Can you work these out from the model? Positions are in its coordinate system, mm. A direction names the side the tool comes from. Give positions to 0.01 mm unless a question says otherwise; leave off trailing zeros. Order: outer loops, then holes, each group sorted by start corner. A loop starts at its lowest first (then second) coordinate and runs counter-clockwise, first axis right, second up.
Item 1: I'm going to push flat-ended pins straight in: pin 1 Ø2.5 at (x, y) = (86, -43) entering from +Z; pin 2 Ø6.5 at (x, y) = (-95.5, 14.5) entering from +Z; pin 3 Ø1.5 at (x, z) = (30, 2) entering from -Y; pin 4 Ø1.8 at (x, y) = (30, -20) entering from +Z. Where does each tip first touch, or does it pass through?
Item 2: Which directions (+Z, -Z, +X, -X, +Y, -Y) give clear straight access to the entire face, cutting with the end or side of a thin tool? Please do faces 1 (the flat face through (-1, 1, 5)), 2 (the cylindrical face through (-81.095, 45.867, 3.479)), 3 (the flat face through (-47, -35, 3)), 4 (the flat face through (29, -57, 3)), 5 (the cylindrical face through (9.905, -29.867, 1.521)).
Item 3: If I drill on line 1 along X through (y, z) = (29, 1.2); line 2 along Y through (x, z) = (-72, 3.15); line 3 along X through (y, z) = (-15, 3.05), over which ranges is the centre line in solid material (lowest first)?
Item 4: I want a section at A-A, the plane x = -43.5. Write out the boundary of the cut face in (y, z), then the cut area to 3 significant figures.
Item 5: If we mould it in two halves opening along Y, with no side actions, what happens to faces 6 (the flat face through (-40, -60, 2)), 7 (the flat face through (-17, 31, 3)), 8 (the flat face through (70, 60, 2))? For each: +Y half, -Y half, draft (parallel to the pull), parting line (faces both ways), or undercut.
Autodesk Fusion 360 part; units mm, degrees
sketch "Sketch1" plane through (0, 0, 0) normal (0, 0, 1) x (1, 0, 0)
  line L0 (-105, 60) -> (105, 60)
  line L1 (105, 60) -> (105, -60)
  line L2 (105, -60) -> (-105, -60)
  line L3 (-105, -60) -> (-105, 60)
  line L4 (-105, 60) -> (105, -60) construction
  line L5 (105, 60) -> (-105, -60) construction
  dimension "d1" = 210
  dimension "d2" = 120
extrude "Extrude1" add sketch "Sketch1" along normal blind 5
sketch "Sketch2" plane through (0, 0, 5) normal (0, 0, 1) x (1, 0, 0)
  line L0 (-105, -60) -> (105, -60)
  line L1 (105, -60) -> (105, 60)
  line L2 (105, 60) -> (-105, 60)
  line L3 (-105, 60) -> (-105, -60)
  line L4 (0, 60) -> (0, -60) construction
  line L5 (105, 0) -> (-105, 0) construction
  line L6 (-75, 35) -> (-90, 35)
  line L7 (-90, 35) -> (-90, 38)
  line L8 (-90, 38) -> (-75, 38)
  line L9 (-75, 38) -> (-75, 35)
  line L10 (-75, 35) -> (-90, 38) construction
  line L11 (-90, 35) -> (-75, 38) construction
  line L12 (-55, 38) -> (-40, 38)
  line L13 (-40, 38) -> (-40, 35)
  line L14 (-40, 35) -> (-55, 35)
  line L15 (-55, 35) -> (-55, 38)
  line L16 (-55, 38) -> (-40, 35) construction
  line L17 (-40, 38) -> (-55, 35) construction
  line L18 (-40, -38) -> (-40, -35)
  line L19 (-55, -38) -> (-40, -35) construction
  line L20 (-40, -35) -> (-55, -35)
  line L21 (-55, -35) -> (-55, -38)
  line L22 (-55, -38) -> (-40, -38)
  line L23 (-40, -38) -> (-55, -35) construction
  line L24 (-75, -38) -> (-75, -35)
  line L25 (-90, -38) -> (-75, -38)
  line L26 (-90, -35) -> (-75, -38) construction
  line L27 (-75, -35) -> (-90, -38) construction
  line L28 (-75, -35) -> (-90, -35)
  line L29 (-90, -35) -> (-90, -38)
  point P0 (-85, 45)
  point P1 (85, 45)
  point P2 (30, 20)
  point P3 (19, 29)
  point P4 (6, 29)
  point P5 (-17, 29)
  point P6 (-30, 29)
  point P7 (-82.5, 36.5)
  point P8 (-47.5, 36.5)
  point P9 (-82.5, 36.5)
  point P10 (-47.5, 36.5)
  point P11 (-97, 15)
  point P12 (-72, 15)
  point P13 (85, -45)
  point P14 (30, -20)
  point P15 (19, -29)
  point P16 (6, -29)
  point P17 (-17, -29)
  point P18 (-30, -29)
  point P19 (-85, -45)
  point P20 (-97, -15)
  point P21 (-72, -15)
  dimension "d5" = 15
  dimension "d6" = 20
  dimension "d7" = 15
  dimension "d8" = 20
  dimension "d9" = 75
  dimension "d10" = 40
  dimension "d11" = 31
  dimension "d12" = 31
  dimension "d13" = 31
  dimension "d14" = 31
  dimension "d15" = 86
  dimension "d16" = 49
  dimension "d17" = 13
  dimension "d18" = 13
  dimension "d19" = 22.5
  dimension "d20" = 23.5
  dimension "d21" = 35
  dimension "d22" = 23.5
  dimension "d23" = 15
  dimension "d24" = 3
  dimension "d25" = 15
  dimension "d26" = 3
  dimension "d27" = 8
  dimension "d28" = 45
  dimension "d29" = 45
  dimension "d30" = 25
extrude "Extrude2" cut sketch "Sketch2" against normal up to surface (5 mm away) contours L6 L7 L8 L9 | L12 L13 L14 L15 | L18 L20 L21 L22 | L24 L25 L28 L29
hole "Hole1" at (-85, 45, 5) at (85, 45, 5) at (-97, 15, 5) at (-72, 15, 5) at (-72, -15, 5) at (-97, -15, 5) at (-85, -45, 5) at (85, -45, 5) direction (0, 0, -1) diameter 3 depth 5 tip angle 180 counterbore diameter 8 counterbore depth 3
sketch "Sketch3" plane through (0, 0, 0) normal (0, 0, -1) x (-1, 0, 0)
  circle A0 centre (85, -45) radius 1.5
  circle A1 centre (72, -15) radius 1.5
  circle A2 centre (97, 15) radius 1.5
  circle A3 centre (85, 45) radius 1.5
  circle A4 centre (-85, 45) radius 1.5
  circle A5 centre (72, 15) radius 1.5
  circle A6 centre (97, -15) radius 1.5
  circle A7 centre (-85, -45) radius 1.5
  line L0 (75, 35) -> (75, 38)
  line L1 (75, 38) -> (90, 38)
  line L2 (90, 38) -> (90, 35)
  line L3 (90, 35) -> (75, 35)
  line L4 (75, -35) -> (90, -35)
  line L5 (90, -35) -> (90, -38)
  line L6 (90, -38) -> (75, -38)
  line L7 (75, -38) -> (75, -35)
  line L8 (55, 38) -> (55, 35)
  line L9 (55, 35) -> (40, 35)
  line L10 (40, 35) -> (40, 38)
  line L11 (40, 38) -> (55, 38)
  line L12 (55, -35) -> (55, -38)
  line L13 (55, -38) -> (40, -38)
  line L14 (40, -38) -> (40, -35)
  line L15 (40, -35) -> (55, -35)
  line L16 (-105, -60) -> (105, -60)
  line L17 (105, -60) -> (105, 60)
  line L18 (105, 60) -> (-105, 60)
  line L19 (-105, 60) -> (-105, -60)
  point P0 (-19, 29)
  point P1 (-30, 20)
  point P2 (-6, 29)
  point P3 (17, 29)
  point P4 (30, 29)
  point P5 (30, -29)
  point P6 (17, -29)
  point P7 (-6, -29)
  point P8 (-19, -29)
  point P9 (-30, -20)
hole "Hole3" at (-30, 29, 0) at (-17, 29, 0) at (6, 29, 0) at (19, 29, 0) at (30, 20, 0) at (30, -20, 0) at (19, -29, 0) at (6, -29, 0) at (-17, -29, 0) at (-30, -29, 0) direction (0, 0, 1) diameter 3 depth 5 tip angle 180 counterbore diameter 8 counterbore depth 3
sketch "Sketch5" plane through (0, 0, 5) normal (0, 0, 1) x (1, 0, 0)
  line L0 (-105, 60) -> (105, 60)
  line L1 (23.5, 60) -> (35, 60)
  line L2 (35, 60) -> (35, 57)
  line L3 (35, 57) -> (23.5, 57)
  line L4 (23.5, 57) -> (23.5, 60)
  line L5 (105, -60) -> (105, 60)
  line L6 (105, 0) -> (-105, 0)
  line L7 (23.5, -60) -> (35, -60)
  line L8 (23.5, -57) -> (23.5, -60)
  line L9 (35, -57) -> (23.5, -57)
  line L10 (35, -60) -> (35, -57)
  point P0 (35, 60)
  point P1 (105, 60)
  point P2 (23.5, 60)
  dimension "d49" = 70
  dimension "d50" = 11.5
  dimension "d51" = 3
  dimension "d52" = 70
extrude "Extrude3" cut sketch "Sketch5" against normal up to surface (5 mm away)
Results list:
1. pin 1: stops at z = 2
1. pin 2: stops at z = 5
1. pin 3: stops at y = -57
1. pin 4: passes through
2. face 1: +Z, +X, -X, +Y, -Y
2. face 2: +Z
2. face 3: +Z, -Z
2. face 4: +Z, -Z, -Y
2. face 5: -Z
3. line 1: x = -105 to -34, -26 to -21, -13 to 2, 10 to 15, 23 to 105
3. line 2: y = -60 to -19, -11 to 11, 19 to 60
3. line 3: x = -105 to -101, -93 to -76, -68 to 105
4. outline: (-60, 0) - (-38, 0) - (-38, 5) - (-60, 5) - close; (-35, 0) - (35, 0) - (35, 5) - (-35, 5) - close; (38, 0) - (60, 0) - (60, 5) - (38, 5) - close
4. area: 570 mm2
5. face 6: -Y half
5. face 7: undercut
5. face 8: +Y half
